Source: CAD feature listing. Evaluate the final solid. Frame: model axes, mm. A direction names the side the tool comes from. Round coordinates to 2 decimals unless told otherwise and drop trailing zeros. Loops run counter-clockwise (first coordinate to the right, second up) from the corner with the lowest first, then second, coordinate; pieces in that order, holes last. Notation, with made-up numbers: M -15.5,79.5 L 20.5,79.5 A21 cw 20.5,94.5 Z; hole C -26,82.5 d11. An arc over 180 degrees is marked long. One line per item, written item: value.
from build123d import *

# Parameters (mm, degrees)
SKETCH_R        = 2.1
PAD_DEPTH       = 7
SKETCH001_R     = 2.1
PAD001_DEPTH    = 7
SKETCH002_W     = 57
SKETCH002_H     = 27
SKETCH002_R     = 2.1
PAD002_DEPTH    = 7
SKETCH003_R     = 3.6
POCKET_DEPTH    = 2.5
SKETCH004_R     = 3.6
POCKET001_DEPTH = 2
SKETCH005_R     = 3.6
POCKET002_DEPTH = 2
SKETCH006_W     = 42
SKETCH006_H     = 42
SKETCH006_R     = 1.6
SKETCH006_R_2   = 12
PAD003_DEPTH    = 5
SKETCH007_R     = 3.6
POCKET003_DEPTH = 2.5
SKETCH008_R     = 2.1
PAD004_DEPTH    = 0.2
CHAMFER_SIZE    = 3.9
FILLET_R        = 5
FILLET001_R     = 2
FILLET002_R     = 5
FILLET003_R     = 5
FILLET004_R     = 5


with BuildPart() as part:
    # Sketch → Pad (new body)
    with BuildSketch(Plane.XY):
        Polygon((-40, 10), (-40, -10), (-3, -40), (17, -40), (17, 10), align=None)
        Circle(SKETCH_R, mode=Mode.SUBTRACT)
        with Locations((0, -30)):
            Circle(SKETCH_R, mode=Mode.SUBTRACT)
        with Locations((-30, 0)):
            Circle(SKETCH_R, mode=Mode.SUBTRACT)
    extrude(amount=PAD_DEPTH)

    # Sketch001 → Pad001 (new body)
    with BuildSketch(Plane.YZ.offset(17)):
        Polygon((10, 0), (10, -50), (-10, -50), (-40, -20), (-40, 0), align=None)
        with Locations((0, -10)):
            Circle(SKETCH001_R, mode=Mode.SUBTRACT)
        with Locations((0, -40)):
            Circle(SKETCH001_R, mode=Mode.SUBTRACT)
        with Locations((-30, -10)):
            Circle(SKETCH001_R, mode=Mode.SUBTRACT)
    extrude(amount=-PAD001_DEPTH)

    # Sketch002 → Pad002 (new body)
    with BuildSketch(Plane(origin=(0, 10, 0), x_dir=(-1, 0, 0), z_dir=(0, 1, 0))):
        with Locations((11.5, -6.5)):
            Rectangle(SKETCH002_W, SKETCH002_H)
        with Locations((30, -10)):
            Circle(SKETCH002_R, mode=Mode.SUBTRACT)
    extrude(amount=PAD002_DEPTH)

    # Sketch003 → Pocket (cut)
    with BuildSketch(Plane.XY.offset(7)):
        Circle(SKETCH003_R)
        with Locations((-30, 0)):
            Circle(SKETCH003_R)
        with Locations((0, -30)):
            Circle(SKETCH003_R)
    extrude(amount=-POCKET_DEPTH, mode=Mode.SUBTRACT)

    # Sketch004 → Pocket001 (cut)
    with BuildSketch(Plane(origin=(-40, 0, 0), x_dir=(0, -1, 0), z_dir=(-1, 0, 0))):
        with Locations((-30, -10)):
            Circle(SKETCH004_R)
        with Locations((0, -10)):
            Circle(SKETCH004_R)
        with Locations((0, -40)):
            Circle(SKETCH004_R)
    extrude(amount=-POCKET001_DEPTH, mode=Mode.SUBTRACT)

    # Sketch005 → Pocket002 (cut)
    with BuildSketch(Plane(origin=(0, 17, 0), x_dir=(-1, 0, 0), z_dir=(0, 1, 0))):
        with Locations((30, -10)):
            Circle(SKETCH005_R)
    extrude(amount=-POCKET002_DEPTH, mode=Mode.SUBTRACT)

    # Sketch006 → Pad003 (new body)
    with BuildSketch(Plane(origin=(0, 17, 0), x_dir=(-1, 0, 0), z_dir=(0, 1, 0))):
        with Locations((0, 28)):
            Rectangle(SKETCH006_W, SKETCH006_H)
        with Locations((-15.5, 43.5)):
            Circle(SKETCH006_R, mode=Mode.SUBTRACT)
        with Locations((15.5, 43.5)):
            Circle(SKETCH006_R, mode=Mode.SUBTRACT)
        with Locations((15.5, 12.5)):
            Circle(SKETCH006_R, mode=Mode.SUBTRACT)
        with Locations((-15.5, 12.5)):
            Circle(SKETCH006_R, mode=Mode.SUBTRACT)
        with Locations((0, 28)):
            Circle(SKETCH006_R_2, mode=Mode.SUBTRACT)
    extrude(amount=-PAD003_DEPTH)

    # Sketch007 → Pocket003 (cut)
    with BuildSketch(Plane.YZ.offset(17)):
        with Locations((-30, -10)):
            Circle(SKETCH007_R)
        with Locations((0, -10)):
            Circle(SKETCH007_R)
        with Locations((0, -40)):
            Circle(SKETCH007_R)
    extrude(amount=-POCKET003_DEPTH, mode=Mode.SUBTRACT)

    # Sketch008 → Pad004 (new body)
    with BuildSketch(Plane(origin=(0, 15, 0), x_dir=(-1, 0, 0), z_dir=(0, 1, 0))):
        with Locations((30, -10)):
            Circle(SKETCH008_R)
    extrude(amount=-PAD004_DEPTH)

    # Chamfer
    chamfer_edges = [part.edges().sort_by_distance(p)[0] for p in [
        (21, 14.5, 7),
    ]]
    chamfer(chamfer_edges, length=CHAMFER_SIZE)

    # Fillet
    fillet_edges = [part.edges().sort_by_distance(p)[0] for p in [
        (21, 14.5, 49),
        (-21, 14.5, 49),
    ]]
    fillet(fillet_edges, radius=FILLET_R)

    # Fillet001
    fillet001_edges = [part.edges().sort_by_distance(p)[0] for p in [
        (-21, 14.5, 7),
    ]]
    fillet(fillet001_edges, radius=FILLET001_R)

    # Fillet002
    fillet002_edges = [part.edges().sort_by_distance(p)[0] for p in [
        (13.5, 10, -50),
        (-40, 13.5, -20),
    ]]
    fillet(fillet002_edges, radius=FILLET002_R)

    # Fillet003
    fillet003_edges = [part.edges().sort_by_distance(p)[0] for p in [
        (13.5, -40, -20),
        (-3, -40, 3.5),
        (-40, -10, 3.5),
        (13.5, -10, -50),
    ]]
    fillet(fillet003_edges, radius=FILLET003_R)

    # Fillet004
    fillet004_edges = [part.edges().sort_by_distance(p)[0] for p in [
        (21, 14.5, 10.9),
    ]]
    fillet(fillet004_edges, radius=FILLET004_R)


solid = part.part
1. Ray query, line 1 (Z direction, x = 15.5, y = 0); line 2 (Z direction, x = 7, y = -29.5); line 3 (Y direction, x = -30, z = 6). Return the intervals inside material, ascending. Write a range as [from, to].
Report:
line 1: z = [-50, -43.6], [-36.4, -13.6], [-6.4, 7]
line 2: z = [0, 7]
line 3: y = [-18.11, -3.6], [3.6, 17]
2. Section query A-A (x = 0). Return the cut outline in (y, z), and give its area (3 significant figures).
Report:
outline: M -40,0 L -32.1,0 L -32.1,4.5 L -33.6,4.5 L -33.6,7 L -40,7 Z; M -27.9,0 L -2.1,0 L -2.1,4.5 L -3.6,4.5 L -3.6,7 L -26.4,7 L -26.4,4.5 L -27.9,4.5 Z; M 2.1,0 L 10,0 L 10,-20 L 17,-20 L 17,16 L 12,16 L 12,7 L 3.6,7 L 3.6,4.5 L 2.1,4.5 Z; M 12,40 L 17,40 L 17,49 L 12,49 Z
area: 555 mm2
3. Pull-direction query (X, two-part tool) for faces 4 (the face through (-26.566, 1.081, 5.768)), 5 (the face through (-39.527, -9.74, 3.549)), 6 (the face through (18.3, 14.5, 8.2)); classes: released by +X, released by -X, zero draft, split by the parting line, or undercut.
Report:
face 4: undercut
face 5: released by -X
face 6: released by +X
4. Section query C-C (z = -40). Return the cut outline in (x, y), and give its area (3 significant figures).
Report:
outline: M 10,-20 L 17,-20 L 17,-3.6 L 14.5,-3.6 L 14.5,-2.1 L 10,-2.1 Z; M 10,2.1 L 14.5,2.1 L 14.5,3.6 L 17,3.6 L 17,10 L 10,10 Z
area: 173 mm2
5. Reachability of faces 1 (the face through (-10, -9, 0)), 2 (the face through (3.434, 1.081, 5.768)), 3 (the face through (15.77, -0.47, -36.43)) from +Z, -Z, +X, -X, +Y, -Y: full face, straight path, thin tool, end or side. Return the list, or none.
Report:
face 1: -Z, -X, -Y
face 2: +Z
face 3: +X
6. Pin query (flat end, axial travel): pin 1 (6 mm diameter, centred on y = -20, z = -5.5, fed in from -X); pin 2 (10 mm diameter, centred on x = -24, y = -15, fed in from -Z); pin 3 (5 mm diameter, centred on x = -30, z = -10, fed in from -Y); pin 4 (12 mm diameter, centred on x = -0.5, y = 7, fed in from +Z). Return the tip coordinate at first contact, or that it passes through.
Report:
pin 1: stops at x = 10
pin 2: stops at z = 0
pin 3: stops at y = 10
pin 4: stops at z = 49
7. Section query D-D (x = -30). Return the cut outline in (y, z).
Report:
outline: M -18.11,0 L -2.1,0 L -2.1,4.5 L -3.6,4.5 L -3.6,7 L -18.11,7 Z; M 2.1,0 L 10,0 L 10,-7.9 L 14.8,-7.9 L 14.8,-12.1 L 10,-12.1 L 10,-20 L 17,-20 L 17,-13.6 L 15,-13.6 L 15,-6.4 L 17,-6.4 L 17,7 L 3.6,7 L 3.6,4.5 L 2.1,4.5 Z
8. Section query B-B (z = -10). Count the separate pieces of the cut face and the enclosed holes in it, and give its area (3 significant figures).
Report:
separate pieces: 3
enclosed holes: 0
area: 641 mm2
